Here's how the part is built. I have some questions about the finished solid (model axes, mm). Face numbers are marked on the shaded views. A direction names the side the tool comes from. Coordinates: 2 decimals unless noted, no trailing zeros. Write each loop counter-clockwise with the first axis right and the second up, starting at its lowest first coordinate (ties: lowest second). Pieces come first, ordered by that corner, then holes. Notation, with made-up numbers: (16.5, -5.75) - (49.5, -5.75) arc R19 ccw to (49.5, 5.25) - close; hole circle Ø4 at (16.5, -35.75). An arc over 180 degrees is marked (long way). Answer in a Markdown table with one row per item. Add a question column.
Item 1: Imagine slicing it at C-C (x = 7). Please give me the cut outline in (y, z) (3 decimals), plus the area to 3 significant figures.
Item 2: I'm going to push flat-ended pins straight in: pin 1 (1.3 mm diameter, centred on x = -14, z = 0, fed in from -Y); pin 2 (3 mm diameter, centred on x = 13, z = -10.5, fed in from +Y); pin 3 (1.9 mm diameter, centred on x = 0, y = 28, fed in from -Z) (3 decimals). Where does each tip first touch, or does it pass through?
Item 3: If I drill on probe 1 along Z at (x, y) = (10.5, 13) (3 decimals); probe 2 along X at (y, z) = (35, -16.45); probe 3 along Z at (x, y) = (-14, 1) (3 decimals), over which ranges is the centre line in solid material (lowest first)? Write a range as from..to.
Item 4: Imagine slicing it at A-A (y = 7). Please give me the cut outline in (x, z) (3 decimals).
Item 5: Imagine slicing it at B-B (z = 0). Please give me the cut outline in (x, y).
Item 6: Imagine slicing it at D-D (x = -14). Please give me the cut outline in (y, z) (3 decimals).
Item 7: Which directions (+Z, -Z, +X, -X, +Y, -Y) give clear straight access to the entire face, cutting with the end or side of a thin tool? Please do the marked faces 1 and 2.
Autodesk Inventor part; units mm, degrees
ref_plane "YZ Plane" through (0, 0, 0) normal (1, 0, 0) x (0, 1, 0)
ref_plane "XZ Plane" through (0, 0, 0) normal (0, 1, 0) x (-1, 0, 0)
ref_plane "XY Plane" through (0, 0, 0) normal (0, 0, 1) x (1, 0, 0)
sketch "Sketch1" plane through (0, 0, 0) normal (0, 1, 0) x (-1, 0, 0)
  line L0 (20, -15.715) -> (-20, -15.715)
  line L1 (-20, -15.715) -> (-20, 15.715)
  line L2 (-20, 15.715) -> (20, 15.715)
  line L3 (20, 15.715) -> (20, -15.715)
  point P0 (0, 0)
  dimension "d0" = 40
  dimension "d1" = 20
  dimension "d2" = 31.43
  dimension "d3" = 15.715
extrude "Plate1" add sketch "Sketch1" along normal blind 1.5
sketch "Sketch2" plane through (20, 0, 17.215) normal (0, 0, -1) x (-1, 0, 0)
  line L0 (40, 0) -> (0, 0)
  line L1 (0, 0) -> (0, 45)
  line L2 (0, 45) -> (40, 45)
  line L3 (40, 45) -> (40, 0)
edge flange "Flange1" height 45 angle 90 thickness 1.5 bend radius 0.31 thickness toward (0, 0, -1) relief tear relief width 1.5 relief depth 0.75 edges at (0, 1.5, 15.715) wall of the first edge with corners at (-20, 0, 17.215) (20, 0, 17.215) (20, 45, 17.215) (-20, 45, 17.215)
bend "Bend1"
corner "Corner1"
sketch "Sketch3" plane through (-20, 0, -17.215) normal (0, 0, 1) x (1, 0, 0)
  line L0 (40, 0) -> (0, 0)
  line L1 (0, 0) -> (0, 45)
  line L2 (0, 45) -> (40, 45)
  line L3 (40, 45) -> (40, 0)
edge flange "Flange2" height 45 angle 90 thickness 1.5 bend radius 0.31 thickness toward (0, 0, 1) relief tear relief width 1.5 relief depth 0.75 edges at (0, 1.5, -15.715) wall of the first edge with corners at (20, 0, -17.215) (-20, 0, -17.215) (-20, 45, -17.215) (20, 45, -17.215)
bend "Bend2"
corner "Corner2"
sketch "Sketch4" plane through (-20, 45, 17.215) normal (0, 0, 1) x (1, 0, 0)
  line L0 (0, -43.19) -> (0, 0)
  line L1 (0, 0) -> (40, 0)
  line L2 (40, 0) -> (40, -43.19)
  line L3 (0, -43.19) -> (40, -43.19)
  arc A0 (28.9876, -5.6156) -> (11.0124, -5.6156) centre (20, -10) ccw
  line L4 (0, -38.19) -> (40, -38.19)
  line L5 (40, -38.19) -> (40, -28.19)
  line L6 (40, -28.19) -> (0, -28.19)
  line L7 (0, -28.19) -> (0, -38.19)
  line L8 (40, -28.19) -> (28.9876, -5.6156)
  line L9 (11.0124, -5.6156) -> (0, -28.19)
  point P0 (0, -28.19)
  point P1 (20, 0)
  point P2 (40, -28.19)
  dimension "d50" = 10
  dimension "d51" = 20
  dimension "d52" = 20
  dimension "d53" = 38.19
  dimension "d54" = 10
  dimension "d55" = 40
  dimension "d56" = 40
extrude "Extrusion1" cut sketch "Sketch4" against normal blind 50 contours L0 L1 A0 L9 | L8 A0 L1 L2
sketch "Sketch6" plane through (-20, 1.81, 17.215) normal (0, 0, 1) x (1, 0, 0)
  arc A0 (28.9876, 37.5744) -> (11.0124, 37.5744) centre (20, 33.19) ccw
  point P0 (20, -1.81)
hole "Hole2" at (0, 35, 17.215) direction (0, 0, -1) diameter 5 depth 1.5
sketch "Sketch7" plane through (-20, 1.81, -15.715) normal (0, 0, 1) x (1, 0, 0)
  arc A0 (28.9876, 37.5744) -> (11.0124, 37.5744) centre (20, 33.19) ccw
  point P0 (20, -1.81)
hole "Hole3" at (0, 35, -15.715) direction (0, 0, -1) diameter 5.2 depth 1.5
sketch "Sketch8" plane through (0, 1.5, 0) normal (0, 1, 0) x (1, 0, 0)
  line L0 (20, 15.405) -> (20, -15.405)
  line L1 (20, -15.715) -> (-20, -15.715)
  line L2 (-20, -15.405) -> (20, -15.405)
  line L3 (20, 15.405) -> (-20, 15.405)
  point P0 (0, 0)
  point P1 (14, -9.405)
  point P2 (-14, -9.405)
  point P3 (14, 0)
  point P4 (-14, 0)
  point P5 (14, 9.405)
  point P6 (-14, 9.405)
  dimension "d71" = 6
  dimension "d73" = 6
  dimension "d76" = 28
  dimension "d79" = 9.405
hole "Hole4" at (14, 1.5, 9.405) at (-14, 1.5, 9.405) at (14, 1.5, 0) at (-14, 1.5, 0) at (14, 1.5, -9.405) at (-14, 1.5, -9.405) direction (0, -1, 0) diameter 2.1 depth 1.5
sketch "Sketch9" plane through (20, 1.81, -17.215) normal (0, 0, -1) x (-1, 0, 0)
  arc A0 (28.9876, 37.5744) -> (11.0124, 37.5744) centre (20, 33.19) ccw
  circle A1 centre (20, 40.19) radius 1.05
  circle A2 centre (13, 33.19) radius 1.05
  circle A3 centre (20, 26.19) radius 1.05
  circle A4 centre (27, 33.19) radius 1.05
  point P0 (20, -1.81)
  dimension "d89" = 7
  dimension "d90" = 0
  dimension "d91" = 2.1
  dimension "d94" = 360
hole "Hole5" at (0, 28, -17.215) at (7, 35, -17.215) at (-7, 35, -17.215) at (0, 42, -17.215) direction (0, 0, 1) diameter 2.1 depth 1.5
equation "\"d62\" = Thickness"
equation "\"d69\" = Thickness"
equation "\"d87\" = Thickness"
equation "\"d101\" = Thickness"
equation "\"d4\" = Thickness"
equation "\"d5\" = BendReliefWidth"
equation "\"d6\" = BendReliefDepth"
equation "\"d7\" = MinimumRemnant"
equation "\"d8\" = TransitionRadius"
equation "\"d11\" = BendRadius"
equation "\"d12\" = CornerReliefSize"
equation "\"d13\" = GapSize"
equation "\"d14\" = JacobiRadiusSize"
equation "\"d15\" = BendReliefWidth"
equation "\"d16\" = BendReliefDepth"
equation "\"d17\" = MinimumRemnant"
equation "\"d18\" = TransitionRadius"
equation "\"d21\" = BendRadius"
equation "\"d22\" = CornerReliefSize"
equation "\"d23\" = GapSize"
equation "\"d24\" = JacobiRadiusSize"
equation "\"BendReliefWidth\" = Thickness"
equation "\"BendReliefDepth\" = 0.5 * Thickness"
equation "\"CornerReliefSize\" = 4 * Thickness"
equation "\"MinimumRemnant\" = 2 * Thickness"
equation "\"TransitionRadius\" = BendRadius"
equation "\"JacobiRadiusSize\" = BendRadius"
equation "\"GapSize\" = Thickness"
properties part number "axis_12_bottom_frame(top)" material "Aluminum 6061-AHC"
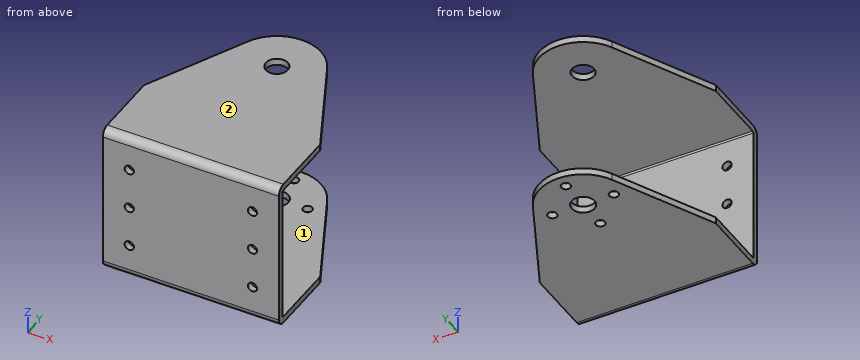
Here are the results:
| question | item | result |
|---|---|---|
| 1 | outline | (0, -15.405) arc R1.81 ccw to (1.81, -17.215) - (33.95, -17.215) - (33.95, -15.715) - (1.81, -15.715) arc R0.31 cw to (1.5, -15.405) - (1.5, 15.405) arc R0.31 cw to (1.81, 15.715) - (42.141, 15.715) - (42.141, 17.215) - (1.81, 17.215) arc R1.81 ccw to (0, 15.405) - close; (36.05, -17.215) - (42.141, -17.215) - (42.141, -15.715) - (36.05, -15.715) - close |
| 1 | area | 169 mm2 |
| 2 | pin 1 | passes through |
| 2 | pin 2 | stops at y = 1.5 |
| 2 | pin 3 | stops at z = 15.715 |
| 3 | probe 1 | z = -17.215..-15.715, 15.715..17.215 |
| 3 | probe 2 | x = -11.13..-8.05, -5.95..-2.6, 2.6..5.95, 8.05..11.13 |
| 3 | probe 3 | z = -17.024..-10.455, -8.355..-1.05, 1.05..8.355, 10.455..17.024 |
| 4 | outline | (-20, -17.215) - (20, -17.215) - (20, -15.715) - (-20, -15.715) - close; (-20, 15.715) - (20, 15.715) - (20, 17.215) - (-20, 17.215) - close |
| 5 | outline | (-20, 0) - (-15.05, 0) - (-15.05, 1.5) - (-20, 1.5) - close; (-12.95, 0) - (12.95, 0) - (12.95, 1.5) - (-12.95, 1.5) - close; (15.05, 0) - (20, 0) - (20, 1.5) - (15.05, 1.5) - close |
| 6 | outline | (0, -15.405) arc R1.81 ccw to (1.81, -17.215) - (29.109, -17.215) - (29.109, -15.715) - (1.81, -15.715) arc R0.31 cw to (1.5, -15.405) - (1.5, -10.455) - (0, -10.455) - close; (0, -8.355) - (1.5, -8.355) - (1.5, -1.05) - (0, -1.05) - close; (0, 1.05) - (1.5, 1.05) - (1.5, 8.355) - (0, 8.355) - close; (0, 10.455) - (1.5, 10.455) - (1.5, 15.405) arc R0.31 cw to (1.81, 15.715) - (29.109, 15.715) - (29.109, 17.215) - (1.81, 17.215) arc R1.81 ccw to (0, 15.405) - close |
| 7 | face 1 | +X, -X, +Y |
| 7 | face 2 | +Z, +X, -X, +Y, -Y |
